CAD build for the part. Positions are in the model's coordinates, mm. Face numbers are marked on the shaded views. A direction names the side the tool comes from. Coordinates: 2 decimals unless noted, no trailing zeros. Order: outer loops, then holes, each group sorted by start corner. A loop starts at its lowest first (then second) coordinate and runs counter-clockwise, first axis right, second up. Notation, with made-up numbers: (-10.5, 87) - (48.5, 87) arc R5 ccw to (48.5, 94) - close; hole circle Ø4 at (-38, 80.25). An arc over 180 degrees is marked (long way). Write each question's results on one line, items separated by ' | '. Start each with the question number.
Q1. Band-saw the part on C-C, the plane y = 2. Write the cut outline in (x, z).
Q2. Wall check: probe 1 along Z at (x, y) = (4, -3); probe 2 along Z at (x, y) = (-6.5, -1.25); probe 3 along X at (y, z) = (0.5, -52.5). Give the ranges that are in metal, low to high.
Q3. Pull direction Z, two halves, no side cores. Call the marked faces 3, 4 and 5: released by +Z, released by -Z, zero draft, split by the parting line, or undercut.
Q4. Band-saw the part on D-D, the plane z = 16.5. Write the cut outline in (x, y), then the cut area to 3 significant figures.
Q5. Band-saw the part on B-B, the plane z = -48.5. Write the cut outline in (x, y).
Q6. Pin check, flat tips, straight feed: P1, Ø2.5, axis at x = -0.5, z = -52, coming from the -Y side; P2, Ø1, axis at y = 1, z = 11, coming from the +X side; P3, Ø5, axis at y = 3.5, z = -3.5, coming from the +X side; P4, Ø2, axis at x = 3.5, y = 0.5, coming from the -Z side. Stop position of each tip, or through.
Q7. Band-saw the part on A-A, the plane x = 0. Write the cut outline in (y, z), then the cut area to 3 significant figures.
Q8. Which spindle directions (+Z, -Z, +X, -X, +Y, -Y) get a long thin tool onto all of the face, cutting with end or side? Do the marked faces 1 and 2. Say none if no direction does.
```python
from build123d import *

# Parameters (mm, degrees)
BOSS_EXTRUDE1_DEPTH = 27
SKETCH2_R           = 4.5
BOSS_EXTRUDE2_DEPTH = 61
CUT_EXTRUDE1_DEPTH  = 14
SKETCH4_R           = 6
BOSS_EXTRUDE3_DEPTH = 33
BOSS_EXTRUDE4_DEPTH = 6.51


with BuildPart() as part:
    # Sketch1 → Boss-Extrude1 (new body)
    with BuildSketch(Plane.XY):
        Polygon((3.666174209, -6.35), (7.332348419, 0), (3.666174209, 6.35), (-3.666174209, 6.35), (-7.332348419, 0), (-3.666174209, -6.35), align=None)
    extrude(amount=BOSS_EXTRUDE1_DEPTH)

    # Sketch2 → Boss-Extrude2 (add)
    with BuildSketch(Plane(origin=(0, 0, 0), x_dir=(-1, 0, 0), z_dir=(0, 0, -1))):
        with Locations(Location((0, 0, 0), (0, 0, 180))):
            Circle(SKETCH2_R)
    extrude(amount=BOSS_EXTRUDE2_DEPTH)

    # Sketch3 → Cut-Extrude1 (cut)
    with BuildSketch(Plane(origin=(0, 0, -61), x_dir=(-1, 0, 0), z_dir=(0, 0, -1))):
        with BuildLine():
            Line((-2.645751311, 3), (2.645751311, 3))
            ThreePointArc((2.645751311, 3), (4, 0), (2.645751311, -3))
            Line((2.645751311, -3), (-2.645751311, -3))
            ThreePointArc((-2.645751311, -3), (-4, 0), (-2.645751311, 3))
        make_face()
    extrude(amount=-CUT_EXTRUDE1_DEPTH, mode=Mode.SUBTRACT)

    # Sketch4 → Boss-Extrude3 (add)
    with BuildSketch(Plane(origin=(0, 0, -61), x_dir=(-1, 0, 0), z_dir=(0, 0, -1))):
        Circle(SKETCH4_R)
        with BuildLine():
            Line((-2.645751311, -3), (2.645751311, -3))
            ThreePointArc((2.645751311, -3), (4, 0), (2.645751311, 3))
            Line((2.645751311, 3), (-2.645751311, 3))
            ThreePointArc((-2.645751311, 3), (-4, 0), (-2.645751311, -3))
        make_face(mode=Mode.SUBTRACT)
    extrude(amount=-BOSS_EXTRUDE3_DEPTH)

    # Sketch5 → Boss-Extrude4 (add)
    with BuildSketch(Plane.XY.offset(27)):
        Polygon((-3.666174209, 6.35), (-7.332348419, 0), (-3.666174209, -6.35), (3.666174209, -6.35), (7.332348419, 0), (3.666174209, 6.35), align=None)
    extrude(amount=BOSS_EXTRUDE4_DEPTH)


solid = part.part
```
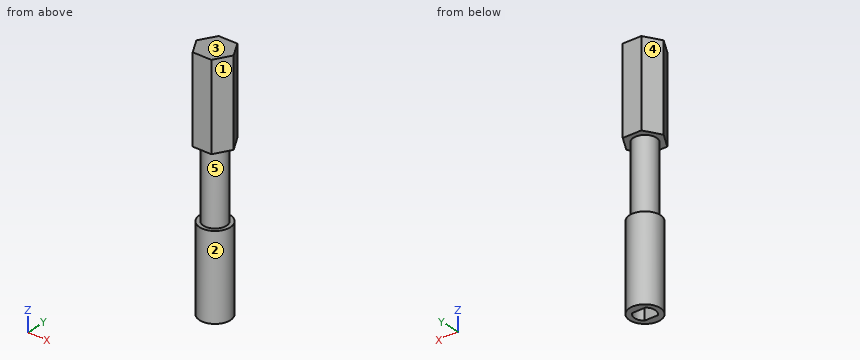
Results below:
1) outline: (-6.18, 0) - (-4.03, 0) - (-4.03, -28) - (-5.66, -28) - (-5.66, -61) - (-3.46, -61) - (-3.46, -47) - (3.46, -47) - (3.46, -61) - (5.66, -61) - (5.66, -28) - (4.03, -28) - (4.03, 0) - (6.18, 0) - (6.18, 33.51) - (-6.18, 33.51) - close
2) probe 1: z = -61 to -28, 0 to 33.51 | probe 2: z = 0 to 33.51 | probe 3: x = -5.98 to -3.97, 3.97 to 5.98
3) face 3: released by +Z | face 4: zero draft | face 5: undercut
4) outline: (-7.33, 0) - (-3.67, -6.35) - (3.67, -6.35) - (7.33, 0) - (3.67, 6.35) - (-3.67, 6.35) - close | area: 140 mm²
5) outline: circle Ø12 at (0, 0); hole (-2.65, -3) - (2.65, -3) arc R4 ccw to (2.65, 3) - (-2.65, 3) arc R4 ccw to start
6) P1: stops at y = -6 | P2: stops at x = 7.04 | P3: stops at x = 4.39 | P4: stops at z = -61
7) outline: (-6.35, 0) - (-4.5, 0) - (-4.5, -28) - (-6, -28) - (-6, -61) - (-3, -61) - (-3, -47) - (3, -47) - (3, -61) - (6, -61) - (6, -28) - (4.5, -28) - (4.5, 0) - (6.35, 0) - (6.35, 33.51) - (-6.35, 33.51) - close | area: 990 mm²
8) face 1: +Z, -Z, +X, -Y | face 2: -Z
